The figure shows three views and two pictorial views of one solid part (mm, origin at its lowest corner). Answer the questions. A direction names the side the tool comes from. Give positions to 0.01 mm unless a question says otherwise; leave off trailing zeros. Loops run counter-clockwise (first coordinate to the right, second up) from the corner with the lowest first, then second, coordinate; pieces in that order, holes last. Notation, with made-up numbers: (52, 8) - (101, 8) arc R27 cw to (101, 39) - close; hole circle Ø2 at (57.5, 30.25). An arc over 180 degrees is marked (long way). One line per question, with ' | ' between items.
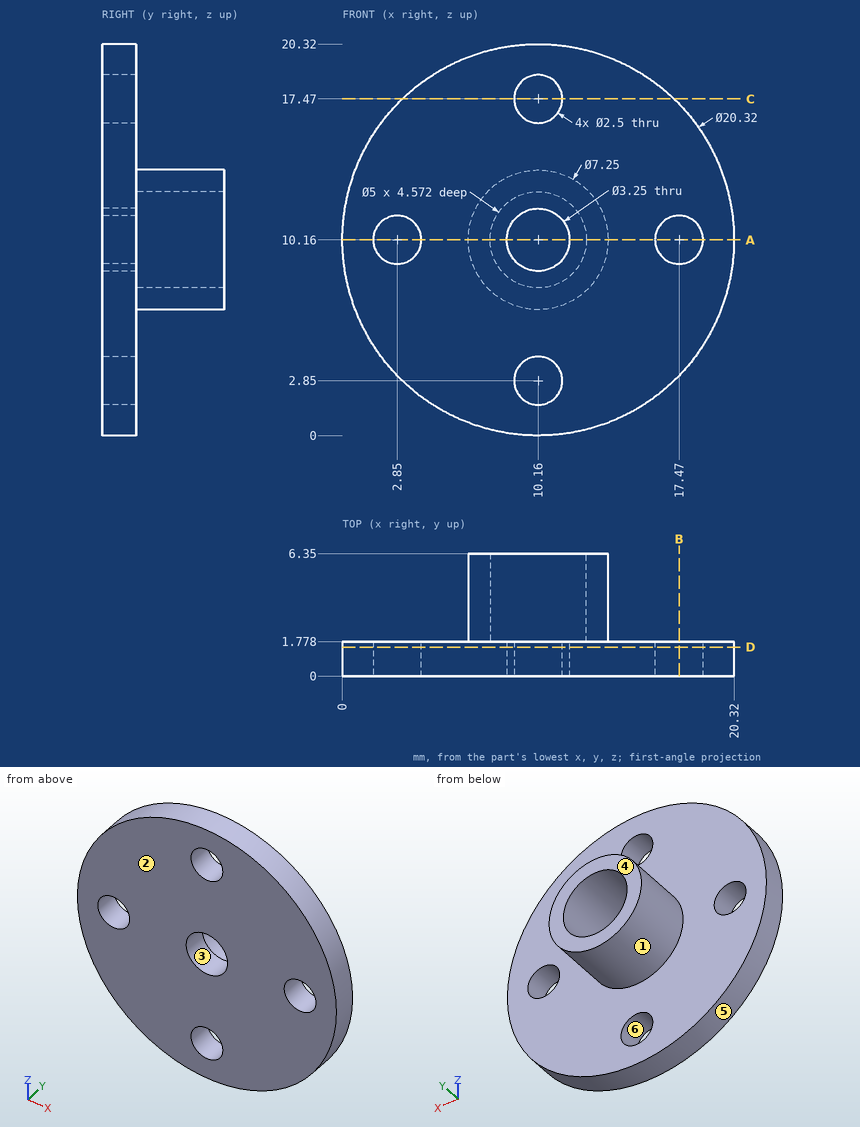
1. Find section D-D on y = 1.5. Write down the section's boundary in (x, z) (3 decimals), then the cut area to 3 significant figures.
Evaluation:
outline: circle Ø20.32 at (10.16, 10.16); hole circle Ø2.5 at (2.85, 10.16); hole circle Ø3.25 at (10.16, 10.16); hole circle Ø2.5 at (10.16, 2.85); hole circle Ø2.5 at (10.16, 17.47); hole circle Ø2.5 at (17.47, 10.16) | area: 296 mm2
2. Which of the six approach directions +Z, -Z, +X, -X, +Y, -Y give full straight-line access (tool end or side, diameter ignored) to the marked faces 1 and 2?
Evaluation:
face 1: +Y | face 2: +Z, -Z, +X, -X, -Y
3. Find section C-C on z = 17.47. Write down the section's boundary in (x, y).
Evaluation:
outline: (3.1, 0) - (8.91, 0) - (8.91, 1.78) - (3.1, 1.78) - close; (11.41, 0) - (17.22, 0) - (17.22, 1.78) - (11.41, 1.78) - close
4. Determine the mould class of the marked faces 3, 4, 5 and 6 for opening direction X: +X half, -X half, draft (parallel to the pull), parting line (faces both ways), or undercut.
Evaluation:
face 3: undercut | face 4: draft | face 5: parting line | face 6: undercut
5. Flat-ended cylindrical pins translate along their axes: pin 1 (1 mm diameter, centred on x = 11.5, y = 5.5, fed in from -Z); pin 2 (4 mm diameter, centred on x = 2.85, z = 10.16, fed in from +Y). Find the tip coordinate at first contact, or state that the pin passes through.
Evaluation:
pin 1: z = 6.63 | pin 2: y = 1.78
6. Find section A-A on z = 10.16. Write down the section's boundary in (x, y) (3 decimals).
Evaluation:
outline: (0, 0) - (1.6, 0) - (1.6, 1.778) - (0, 1.778) - close; (4.1, 0) - (8.535, 0) - (8.535, 1.778) - (7.66, 1.778) - (7.66, 6.35) - (6.535, 6.35) - (6.535, 1.778) - (4.1, 1.778) - close; (11.785, 0) - (16.22, 0) - (16.22, 1.778) - (13.785, 1.778) - (13.785, 6.35) - (12.66, 6.35) - (12.66, 1.778) - (11.785, 1.778) - close; (18.72, 0) - (20.32, 0) - (20.32, 1.778) - (18.72, 1.778) - close
7. Find section B-B on x = 17.47. Write down the section's boundary in (y, z), then the cut area to 3 significant figures.
Evaluation:
outline: (0, 3.1) - (1.78, 3.1) - (1.78, 8.91) - (0, 8.91) - close; (0, 11.41) - (1.78, 11.41) - (1.78, 17.22) - (0, 17.22) - close | area: 20.6 mm2
8. Consider L1, parallel to Z at x = 10.16, y = 0.6 (3 decimals); L2, parallel to Y at x = 1.75, z = 6; L3, parallel to X at y = 4.3, z = 10.16 (3 decimals). Determine where each line is inside the solid, lowest interval first.
Evaluation:
L1: 0 to 1.6, 4.1 to 8.535, 11.785 to 16.22, 18.72 to 20.32 | L2: 0 to 1.78 | L3: 6.535 to 7.66, 12.66 to 13.785
